from build123d import *

# Parameters (mm, degrees)
F0_W     = 20
F0_H     = 20
F1_DEPTH = 16
F2_T     = -2.5


with BuildPart() as f1:
    # F0 (on Front) → F1 (new body)
    with BuildSketch(Plane.XZ):
        Rectangle(F0_W, F0_H)
    extrude(amount=F1_DEPTH)

    # F2
    f2_openings = [f1.faces().sort_by_distance(p)[0] for p in [
        (0, -8, -10),
        (10, -8, 0),
    ]]
    offset(amount=F2_T, openings=f2_openings)


solid = f1.part
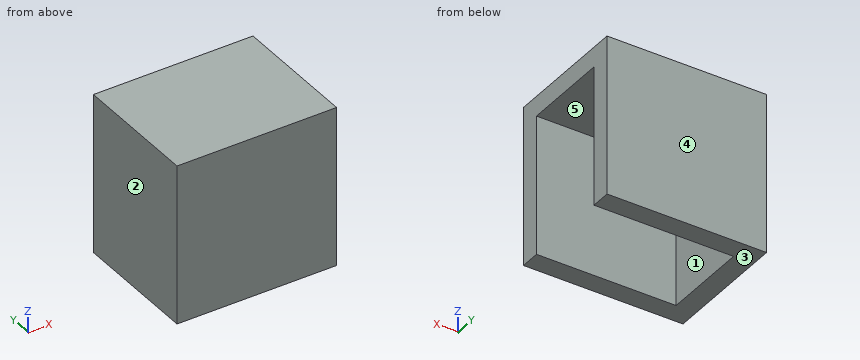
The listing builds one solid part. Answer for the finished solid, in the listing's coordinates (mm). Face numbers are marked on the shaded views. A direction names the side the tool comes from. Give positions to 0.01 mm unless a question says otherwise; leave off trailing zeros. Loops run counter-clockwise (first coordinate to the right, second up) from the corner with the lowest first, then second, coordinate; pieces in that order, holes last. Notation, with made-up numbers: (20, 76) - (67, 76) arc R11 ccw to (67, 84) - close; hole circle Ø11 at (-36, 20.25). An arc over 180 degrees is marked (long way). Write each question's results on one line, items separated by ' | '.
1. Find section B-B, the plane x = -2.25. Write down the section's boundary in (y, z).
Resolved:
outline: (-16, -10) - (-13.5, -10) - (-13.5, 7.5) - (-2.5, 7.5) - (-2.5, -10) - (0, -10) - (0, 10) - (-16, 10) - close
2. Consider probe 1 along Y at (x, z) = (-0.5, -0.5); probe 2 along Z at (x, y) = (7.5, -5.25); probe 3 along X at (y, z) = (-11, 2.5). Determine where each line is inside the solid, lowest interval first. Write a range as from..to.
Resolved:
probe 1: y = -16..-13.5, -2.5..0 | probe 2: z = 7.5..10 | probe 3: x = -10..-7.5
3. Which of the six approach directions +Z, -Z, +X, -X, +Y, -Y give full straight-line access (tool end or side, diameter ignored) to the marked faces 1 and 2?
Resolved:
face 1: -Z, +X | face 2: +Z, -Z, -X, +Y, -Y
4. Flat-ended cylindrical pins translate along their axes: P1, Ø5, axis at y = -11.5, z = 7, coming from the +X side; P2, Ø3.5, axis at x = -1, y = -10.5, coming from the -Z side; P3, Ø4, axis at y = -8, z = -7, coming from the +X side. Find the tip coordinate at first contact, or state that the pin passes through.
Resolved:
P1: stops at x = 10 | P2: stops at z = 7.5 | P3: stops at x = -7.5
5. For a pull along Y with two mould halves and no side action, classify the marked faces 3, 4 and 5 as +Y half, -Y half, draft (parallel to the pull), parting line (faces both ways), or undercut.
Resolved:
face 3: draft | face 4: +Y half | face 5: undercut
6. Find section C-C, the plane y = -4.75. Write down the section's boundary in (x, z).
Resolved:
outline: (-10, -10) - (-7.5, -10) - (-7.5, 7.5) - (10, 7.5) - (10, 10) - (-10, 10) - close
7. Find section A-A, the plane z = 2.75. Write down the section's boundary in (x, y), then the cut area to 4 significant figures.
Resolved:
outline: (-10, -16) - (10, -16) - (10, -13.5) - (-7.5, -13.5) - (-7.5, -2.5) - (10, -2.5) - (10, 0) - (-10, 0) - close | area: 127.5 mm^2
